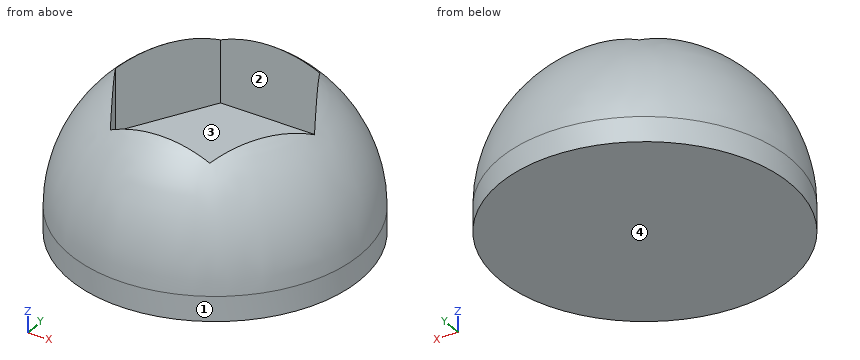
```python
from build123d import *

# Parameters (mm, degrees)
F0_R     = 17.5
F1_DEPTH = 20
F3_DEPTH = 12


# Not quite as in the source:
# - a fillet or chamfer that OpenCascade refuses, or shapes differently, is made with other operations: its cross-section is extruded or revolved along the edge and cut away or added


with BuildPart() as f1:
    # F0 (on Top) → F1 (new body)
    with BuildSketch(Plane.XY):
        Circle(F0_R)
    extrude(amount=F1_DEPTH)

    # F2 (on face) → F3 (cut)
    with BuildSketch(Plane.XY.offset(20)):
        Polygon((6, 10.3923048454), (-6, 10.3923048454), (-12, 0), (-6, -10.3923048454), (6, -10.3923048454), (12, 0), align=None)
    extrude(amount=-F3_DEPTH, mode=Mode.SUBTRACT)

    # F4: fillet of radius 17 on 1 edges, made by hand

    # F4_s1 → F4_t2 (revolve, cut)
    with BuildSketch(Plane.XZ):
        with BuildLine():
            ThreePointArc((17.5, 3), (12.5208152802, 15.0208152802), (0.5, 20))
            Line((0.5, 20), (17.5, 20))
            Line((17.5, 20), (17.5, 3))
        make_face()
    revolve(axis=Axis((0, 0, 20), (0, 0, 1)), mode=Mode.SUBTRACT)


solid = f1.part
```
Here's how the part is built. I have some questions about the finished solid (model axes, mm). Face numbers are marked on the shaded views. Round coordinates to 2 decimals unless told otherwise and drop trailing zeros. Write each loop counter-clockwise with the first axis right and the second up, starting at its lowest first coordinate (ties: lowest second). Pieces come first, ordered by that corner, then holes.
Q1. Please list where these lines run through material, in increasing order: probe 1 along Z at (x, y) = (-8, -4); probe 2 along Y at (x, z) = (3, 15); probe 3 along Y at (x, z) = (3, 12.75).
Q2. If we section it at A-A on z = 2.5: Write out the boundary of the cut face in (x, y), plus the area to 3 significant figures.
Q3. Will these pins go through, and if not, where does the flat tip stop? P1, Ø1.5, axis at y = 1.5, z = 2.5, coming from the +X side; P2, Ø6, axis at x = -12, z = 10, coming from the -Y side; P3, Ø6, axis at x = 8, y = -12, coming from the -Z side; P4, Ø10.5, axis at x = -2.5, y = -2.5, coming from the +Z side.
Q4. If we mould it in two halves opening along X, with no side actions, what happens to the marked faces 1, 2, 3 and 4? For each: +X half, -X half, draft (parallel to the pull), parting line (faces both ways), or undercut.
Answer below:
1. probe 1: z = 0 to 8
1. probe 2: y = -12.18 to -10.39, 10.39 to 12.18
1. probe 3: y = -14.11 to -10.39, 10.39 to 14.11
2. outline: circle Ø35 at (0, 0)
2. area: 962 mm2
3. P1: stops at x = 17.48
3. P2: stops at y = -13.66
3. P3: stops at z = 0
3. P4: stops at z = 8
4. face 1: parting line
4. face 2: undercut
4. face 3: undercut
4. face 4: draft
